For this review, use the dimensioned drawing (mm, ordinates from the lowest corner) and the shaded views. A direction names the side the tool comes from. Give positions to 0.01 mm unless a question says otherwise; leave off trailing zeros. Loops run counter-clockwise (first coordinate to the right, second up) from the corner with the lowest first, then second, coordinate; pieces in that order, holes last. Notation, with made-up numbers: M -4.75,7 L 18.25,7 A27 cw 18.25,33 Z; hole C -11.5,21 d3. An arc over 180 degrees is marked long. Use CSV: the item, a comma, the result in double quotes. Start each with the question number.
1. The part is to be moulded in two halves that separate along X. For the marked faces 5, 6, 7 and 8, say which applies: pulls with the +X half, pulls with the -X half, needs draft (parallel to the pull), parting line crosses it, or undercut.
2. Take a section at A-A, the plane z = 182. Write out the cut boundary in (x, y), and give its area (3 significant figures).
3. Insertion check: P1, Ø10, axis at x = 53, y = 11, coming from the -Z side (3 decimals). The pin has a flat end and moves straight along its axis. Give the tip position at first contact, or say it passes through.
4. Take a section at D-D, the plane y = 8. Write out the cut boundary in (x, z) (3 decimals).
5. Tool access review of the marked faces 1, 2, 3 and 4: name each direction out of +Z, -Z, +X, -X, +Y, -Y from which nothing blocks a thin tool from reaching the whole face with its end or side.
6. Take a section at C-C, the plane x = 54.5. Write out the cut boundary in (y, z) (3 decimals), and give its area (3 significant figures).
7. To check wall thickness, follow line 1 (Z direction, x = 103, y = 33) (3 decimals); line 2 (Z direction, x = 73, y = 36) (3 decimals); line 3 (Z direction, x = 188.5, y = 13.5) (3 decimals). State the ranges of each line that lie inside material, in increasing order. Write a range as [from, to].
8. Take a section at B-B, the plane x = 143.5. Write out the cut boundary in (y, z) (3 decimals), and give its area (3 significant figures).
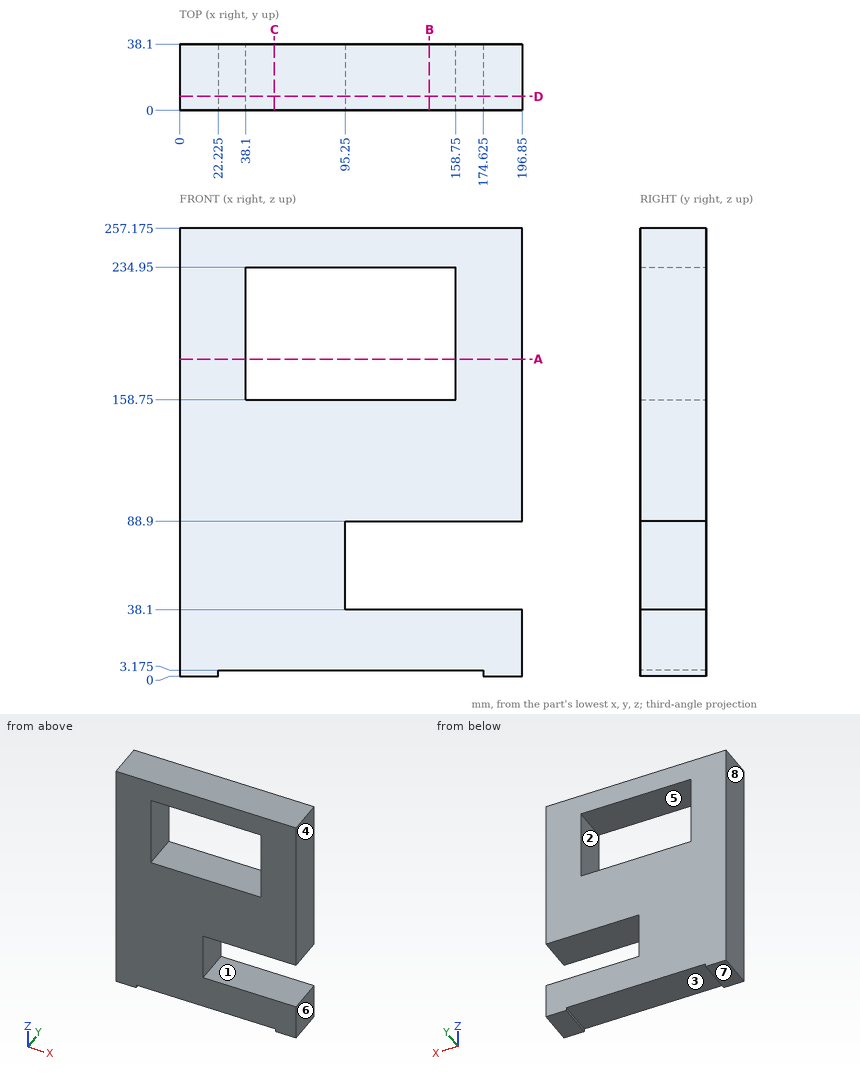
Result set:
1,face 5,"undercut"
1,face 6,"pulls with the +X half"
1,face 7,"needs draft"
1,face 8,"pulls with the -X half"
2,outline,"M 0,0 L 38.1,0 L 38.1,38.1 L 0,38.1 Z; M 158.75,0 L 196.85,0 L 196.85,38.1 L 158.75,38.1 Z"
2,area,"2,900 mm2"
3,P1,"z = 3.175"
4,outline,"M 0,0 L 22.225,0 L 22.225,3.175 L 174.625,3.175 L 174.625,0 L 196.85,0 L 196.85,38.1 L 95.25,38.1 L 95.25,88.9 L 196.85,88.9 L 196.85,257.175 L 0,257.175 Z; hole M 38.1,158.75 L 158.75,158.75 L 158.75,234.95 L 38.1,234.95 Z"
5,face 1,"+X, +Y, -Y"
5,face 2,"+Y, -Y"
5,face 3,"-Z, +Y, -Y"
5,face 4,"+Z, -Z, +X, +Y, -Y"
6,outline,"M 0,3.175 L 38.1,3.175 L 38.1,158.75 L 0,158.75 Z; M 0,234.95 L 38.1,234.95 L 38.1,257.175 L 0,257.175 Z"
6,area,"6,770 mm2"
7,line 1,"[3.175, 38.1], [88.9, 158.75], [234.95, 257.175]"
7,line 2,"[3.175, 158.75], [234.95, 257.175]"
7,line 3,"[0, 38.1], [88.9, 257.175]"
8,outline,"M 0,3.175 L 38.1,3.175 L 38.1,38.1 L 0,38.1 Z; M 0,88.9 L 38.1,88.9 L 38.1,158.75 L 0,158.75 Z; M 0,234.95 L 38.1,234.95 L 38.1,257.175 L 0,257.175 Z"
8,area,"4,840 mm2"
